Study the drawing (mm; zero at the part's minimum x, y, z) and answer. Give positions to 0.01 mm unless a question says otherwise; leave off trailing zeros. Order: outer loops, then holes, each group sorted by start corner. A loop starts at its lowest first (then second) coordinate and runs counter-clockwise, first axis right, second up. Notation, with made-up numbers: (65.5, -3.5) - (112.5, -3.5) arc R16 cw to (112.5, 4.5) - close; hole circle Ø5 at (-40, 38). An arc over 180 degrees is marked (long way). Use CSV: the item, a comma, the result in double quotes.
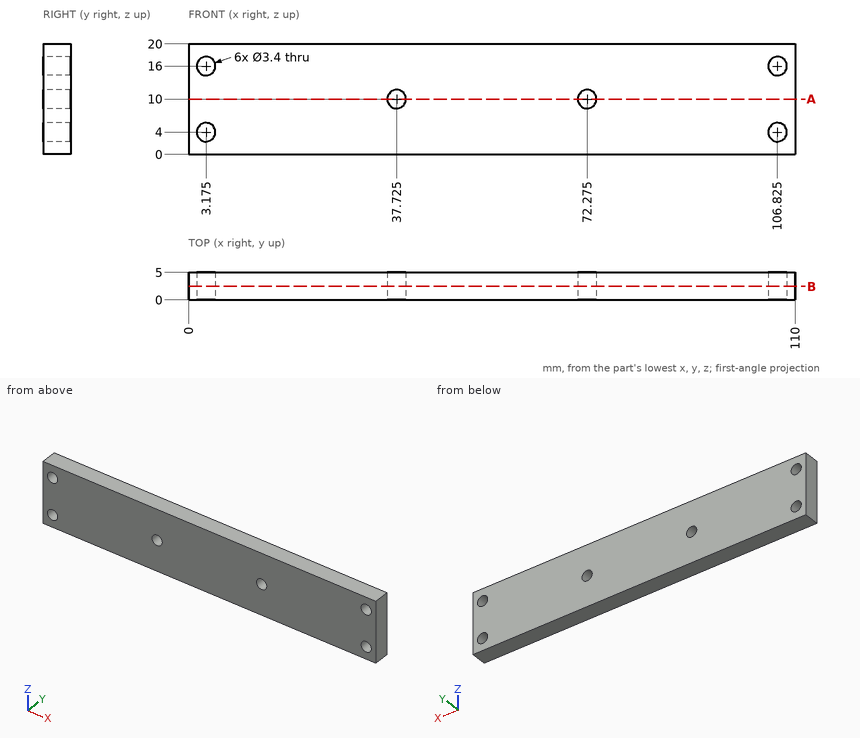
Item 1: The part is cut by section A-A (z = 10). Give the vertices of the cut face in (x, y) (3 decimals).
Taken from the geometry:
outline,"(0, 0) - (36.025, 0) - (36.025, 5) - (0, 5) - close; (39.425, 0) - (70.575, 0) - (70.575, 5) - (39.425, 5) - close; (73.975, 0) - (110, 0) - (110, 5) - (73.975, 5) - close"
Item 2: The part is cut by section B-B (y = 2.45). Give the vertices of the cut face in (x, z) (3 decimals), and give its area (3 significant figures).
Taken from the geometry:
outline,"(0, 0) - (110, 0) - (110, 20) - (0, 20) - close; hole circle Ø3.4 at (3.175, 4); hole circle Ø3.4 at (3.175, 16); hole circle Ø3.4 at (37.725, 10); hole circle Ø3.4 at (72.275, 10); hole circle Ø3.4 at (106.825, 4); hole circle Ø3.4 at (106.825, 16)"
area,"2,150 mm^2"
Item 3: Find the intervals of material crossed by line 1 along X through (y, z) = (1.1, 10) (3 decimals); line 2 along X through (y, z) = (4.35, 16) (3 decimals), in increasing order.
Taken from the geometry:
line 1,"0 to 36.025, 39.425 to 70.575, 73.975 to 110"
line 2,"0 to 1.475, 4.875 to 105.125, 108.525 to 110"
